The listing builds one solid part. Answer for the finished solid, in the listing's coordinates (mm). Round coordinates to 2 decimals unless told otherwise and drop trailing zeros. Write each loop counter-clockwise with the first axis right and the second up, starting at its lowest first coordinate (ties: lowest second). Pieces come first, ordered by that corner, then holes.
Item 1: Each of these flat-tipped pins is pushed along its axis until it touches: pin 1 (2 mm diameter, centred on x = -33.5, z = 1.5, fed in from +Y); pin 2 (6 mm diameter, centred on x = -59, z = 3, fed in from +Y); pin 3 (4 mm diameter, centred on x = -79, z = 4, fed in from -Y). Where does it stop, or does it pass through?
Item 2: Find section B-B on x = -54.5. Give the vertices of the cut face in (y, z).
Item 3: Find the intervals of material crossed by probe 1 along Y at (x, z) = (-15, 4.5); probe 2 along Y at (x, z) = (-99, 1.5); probe 3 along Y at (x, z) = (-100.5, 9.25), in increasing order.
Item 4: For a pull along Y with two mould halves and no side action, classify faces 1 (the face through (-64.187, -25.633, 4.93)), 2 (the face through (-17.406, 26.018, 4.93)), 3 (the face through (0, 0, 5)) as +Y half, -Y half, draft (parallel to the pull), parting line (faces both ways), or undercut.
Item 5: Find section C-C on x = -7.5. Give the vertices of the cut face in (y, z).
Item 6: Find section A-A on z = 7.25. Give the vertices of the cut face in (x, y), then the cut area to 3 significant figures.
```python
from build123d import *

# Parameters (mm, degrees)
SKETCH1_R               = 3.2639
BOSS_EXTRUDE1_DEPTH     = 10
SKETCH2_W               = 55.96454122
SKETCH2_H               = 39.556429901
BOSS_EXTRUDE2_DEPTH     = 50
CUT_EXTRUDE1_DEPTH      = 3.621876658
CUT_EXTRUDE1_DEPTH_BACK = 57.750909587
CUT_EXTRUDE3_DEPTH      = 104.020815944
BOSS_EXTRUDE3_REACH     = 105.021
SKETCH10_R              = 90
CUT_EXTRUDE4_DEPTH      = 50
CUT_EXTRUDE6_DEPTH      = 2.714029404
CUT_EXTRUDE6_DEPTH_BACK = 57.750909587


with BuildPart() as part:
    # Sketch1 → Boss-Extrude1 (new body)
    with BuildSketch(Plane.XY):
        with BuildLine():
            ThreePointArc((0, -23.8125), (-4.393398282, -34.419101718), (-15, -38.8125))
            Line((-15, -38.8125), (-119.778475404, -10.737192131))
            Line((-119.778475404, -10.737192131), (-119.778475404, 66.887807869))
            Line((-119.778475404, 66.887807869), (-15, 38.8125))
            ThreePointArc((-15, 38.8125), (-4.393398282, 34.419101718), (0, 23.8125))
            Line((0, 23.8125), (0, -23.8125))
        make_face()
        with Locations((-15, 23.8125)):
            Circle(SKETCH1_R, mode=Mode.SUBTRACT)
        with Locations((-15, -23.8125)):
            Circle(SKETCH1_R, mode=Mode.SUBTRACT)
    extrude(amount=BOSS_EXTRUDE1_DEPTH)

    # Sketch2 → Boss-Extrude2 (add)
    with BuildSketch(Plane.XY.offset(10)):
        with Locations((-137.760746014, 83.986530895)):
            Rectangle(SKETCH2_W, SKETCH2_H)
    extrude(amount=-BOSS_EXTRUDE2_DEPTH)

    # Sketch4 → Cut-Extrude1 (cut, two sides)
    with BuildSketch(Plane(origin=(-0.959208406, 0, 16.788657247), x_dir=(0, 1, 0), z_dir=(-0.057041289, 0, 0.99837182))) as cut_extrude1_sk:
        with BuildLine():
            ThreePointArc((64.208315944, 114.013041626), (81.708315944, 131.513041626), (64.208315944, 149.013041626))
            Line((64.208315944, 149.013041626), (64.208315944, 176.700065815))
            Line((64.208315944, 176.700065815), (111.984574651, 176.700065815))
            Line((111.984574651, 176.700065815), (111.984574651, 106.901315277))
            Line((111.984574651, 106.901315277), (64.208315944, 106.901315277))
            Line((64.208315944, 106.901315277), (64.208315944, 114.013041626))
        make_face()
        with BuildLine():
            Line((64.208315944, 144.013041626), (64.208315944, 119.013041626))
            ThreePointArc((64.208315944, 119.013041626), (76.708315944, 131.513041626), (64.208315944, 144.013041626))
        make_face()
    extrude(amount=CUT_EXTRUDE1_DEPTH, mode=Mode.SUBTRACT)
    extrude(cut_extrude1_sk.sketch, amount=-CUT_EXTRUDE1_DEPTH_BACK, mode=Mode.SUBTRACT)

    # Sketch7 → Cut-Extrude3 (cut, through all)
    with BuildSketch(Plane(origin=(0, 64.208315944, 0), x_dir=(1, 0, 0), z_dir=(0, 1, 0))):
        Polygon((-119.778475404, 0), (-119.207132269, 0), (-119.778475404, -10), align=None)
    extrude(amount=-CUT_EXTRUDE3_DEPTH, mode=Mode.SUBTRACT)

    # Boss-Extrude3: up to this face of the body (flat: up to its plane)
    boss_extrude3_end = Plane(part.part.faces().sort_by_distance((-67.246532084, -24.813083921, 5.004556479))[0])
    # Sketch8 → Boss-Extrude3 (add, up to the picked face)
    with BuildSketch(Plane.XZ.offset(-64.208315944), mode=Mode.PRIVATE) as boss_extrude3_sk1:
        Polygon((-119.207132269, 0), (-116.92175973, -40), (-111.913605554, -40), (-114.198978093, 0), align=None)
    boss_extrude3_tool1 = split(extrude(boss_extrude3_sk1.sketch, amount=BOSS_EXTRUDE3_REACH, mode=Mode.PRIVATE), bisect_by=boss_extrude3_end, keep=Keep.BOTH, mode=Mode.PRIVATE)
    add(boss_extrude3_tool1.solids().sort_by_distance((-115.560369, 64.208316, -20))[0])

    # Sketch10 → Cut-Extrude4 (cut)
    with BuildSketch(Plane(origin=(-113.827407897, 0, -6.503450805), x_dir=(0.057041289, 0, -0.99837182), z_dir=(0.99837182, 0, 0.057041289))):
        with Locations((83.472510719, -10.677332841)):
            Circle(SKETCH10_R)
    extrude(amount=-CUT_EXTRUDE4_DEPTH, mode=Mode.SUBTRACT)

    # Sketch14 → Cut-Extrude6 (cut, two sides)
    with BuildSketch(Plane(origin=(-0.959208406, 0, 16.788657247), x_dir=(0, 1, 0), z_dir=(-0.057041289, 0, 0.99837182))) as cut_extrude6_sk:
        Polygon((64.208315944, 114.013041626), (103.707100536, 114.013041626), (103.707100536, 158.820530176), (-53.093138129, 158.820530176), (-49.03095578, 114.013041626), align=None)
    extrude(amount=CUT_EXTRUDE6_DEPTH, mode=Mode.SUBTRACT)
    extrude(cut_extrude6_sk.sketch, amount=-CUT_EXTRUDE6_DEPTH_BACK, mode=Mode.SUBTRACT)


solid = part.part
```
Check values:
1. pin 1: stops at y = 44.04
1. pin 2: stops at y = 51.41
1. pin 3: stops at y = -22.2
2. outline: (-28.23, 0) - (49.4, 0) - (49.4, 10) - (-28.23, 10) - close
3. probe 1: y = -38.81 to -27.08, -20.55 to 20.55, 27.08 to 38.81
3. probe 2: y = -16.3 to 61.32
3. probe 3: y = -15.9 to 61.72
4. face 1: -Y half
4. face 2: undercut
4. face 3: draft
5. outline: (-36.8, 0) - (36.8, 0) - (36.8, 10) - (-36.8, 10) - close
6. outline: (-114.61, -12.12) - (-15, -38.81) arc R15 ccw to (0, -23.81) - (0, 23.81) arc R15 ccw to (-15, 38.81) - (-109.78, 64.21) - (-114.61, 64.21) - close; hole circle Ø6.53 at (-15, -23.81); hole circle Ø6.53 at (-15, 23.81)
6. area: 8,730 mm2
